For this review, use the dimensioned drawing (mm, ordinates from the lowest corner) and the shaded views. Give positions to 0.01 mm unless a question says otherwise; leave off trailing zeros. Loops run counter-clockwise (first coordinate to the right, second up) from the corner with the lowest first, then second, coordinate; pieces in that order, holes last. Notation, with made-up numbers: M 34.25,49.25 L 82.25,49.25 A10 cw 82.25,55.25 Z; hole C -32.75,-2.75 d1. An arc over 180 degrees is marked long. Use a Markdown table: item, result. Add a question column.
(1) Add section B-B, the plane x = 50. Give the boundary of the cut face in (y, z), then the cut area to 3 significant figures.
(2) Add section D-D, the plane z = 0.75. State how many separate pieces and enclosed holes the cut face has, then the cut area to 3 significant figures.
(3) Add section A-A, the plane y = 10. Give the boundary of the cut face in (x, z).
(4) For probe 1 along Y at (x, z) = (10, 2.95); probe 2 along Y at (x, z) = (50, 1.8); probe 3 along X at (y, z) = (31.5, 1.4) (1 decimal), list the stretches that pass through material, from the lowest coordinate up.
(5) Add section C-C, the plane y = 70. Give the boundary of the cut face in (x, z).
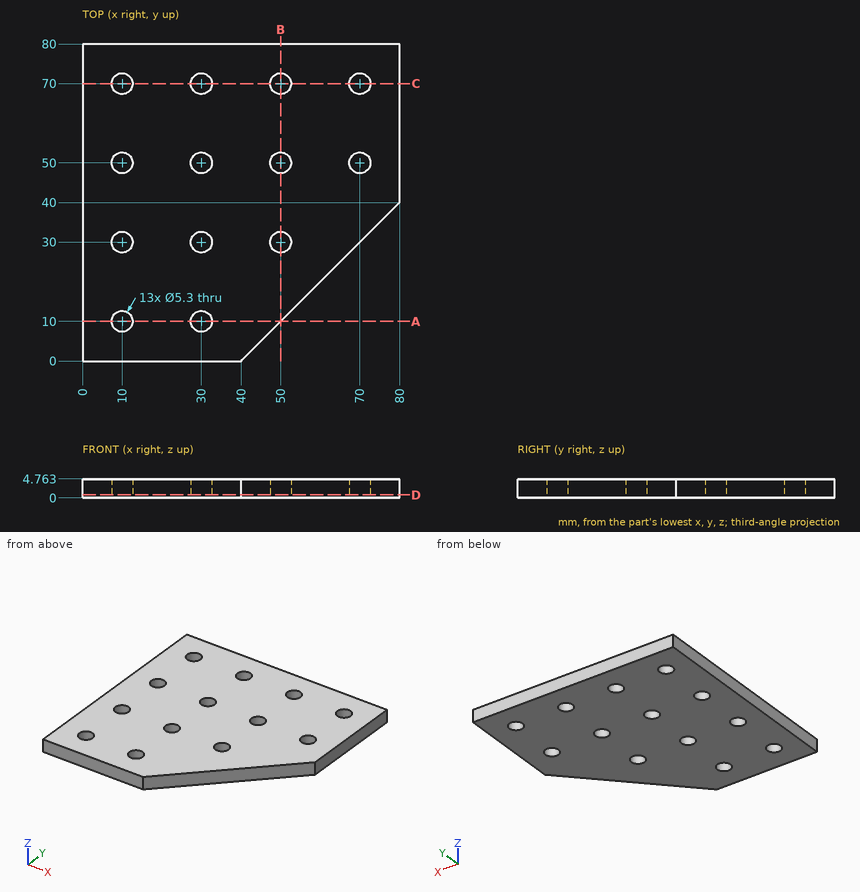
Established:
| question | item | result |
|---|---|---|
| 1 | outline | M 10,0 L 27.35,0 L 27.35,4.76 L 10,4.76 Z; M 32.65,0 L 47.35,0 L 47.35,4.76 L 32.65,4.76 Z; M 52.65,0 L 67.35,0 L 67.35,4.76 L 52.65,4.76 Z; M 72.65,0 L 80,0 L 80,4.76 L 72.65,4.76 Z |
| 1 | area | 258 mm^2 |
| 2 | separate pieces | 1 |
| 2 | enclosed holes | 13 |
| 2 | area | 5,310 mm^2 |
| 3 | outline | M 0,0 L 7.35,0 L 7.35,4.76 L 0,4.76 Z; M 12.65,0 L 27.35,0 L 27.35,4.76 L 12.65,4.76 Z; M 32.65,0 L 50,0 L 50,4.76 L 32.65,4.76 Z |
| 4 | probe 1 | 0 to 7.35, 12.65 to 27.35, 32.65 to 47.35, 52.65 to 67.35, 72.65 to 80 |
| 4 | probe 2 | 10 to 27.35, 32.65 to 47.35, 52.65 to 67.35, 72.65 to 80 |
| 4 | probe 3 | 0 to 7.8, 12.2 to 27.8, 32.2 to 47.8, 52.2 to 71.5 |
| 5 | outline | M 0,0 L 7.35,0 L 7.35,4.76 L 0,4.76 Z; M 12.65,0 L 27.35,0 L 27.35,4.76 L 12.65,4.76 Z; M 32.65,0 L 47.35,0 L 47.35,4.76 L 32.65,4.76 Z; M 52.65,0 L 67.35,0 L 67.35,4.76 L 52.65,4.76 Z; M 72.65,0 L 80,0 L 80,4.76 L 72.65,4.76 Z |
